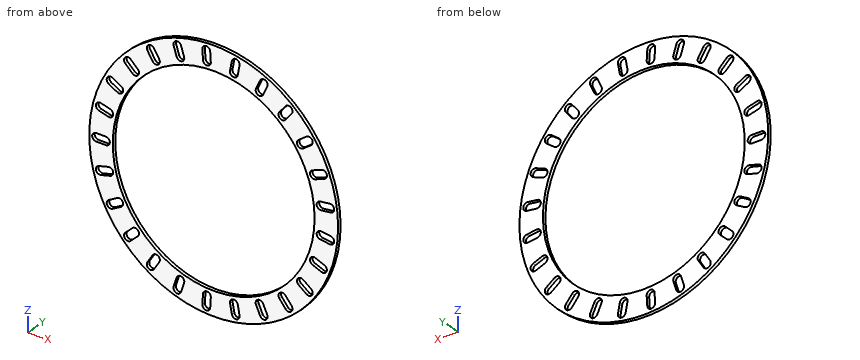
from build123d import *

# Parameters (mm, degrees)
SKETCH1_R           = 31.77
SKETCH1_R_2         = 25.77
BOSS_EXTRUDE1_DEPTH = 0.85
CUT_EXTRUDE1_DEPTH  = 1.85
CIRPATTERN1_COUNT   = 25


with BuildPart() as part:
    # Sketch1 → Boss-Extrude1 (new body)
    with BuildSketch(Plane(origin=(0, 0, 0), x_dir=(1, 0, 0), z_dir=(0, 1, 0))):
        Circle(SKETCH1_R)
        Circle(SKETCH1_R_2, mode=Mode.SUBTRACT)
    extrude(amount=BOSS_EXTRUDE1_DEPTH)

    # Sketch3 → Cut-Extrude1 (cut, through all)
    with BuildSketch(Plane(origin=(0, 0.85, 0), x_dir=(1, 0, 0), z_dir=(0, 1, 0))):
        with BuildLine():
            Line((-30.02, 1), (-27.52, 1))
            ThreePointArc((-27.52, 1), (-26.52, 0), (-27.52, -1))
            Line((-27.52, -1), (-30.02, -1))
            ThreePointArc((-30.02, -1), (-31.02, 0), (-30.02, 1))
        make_face()
    cut_extrude1 = extrude(amount=-CUT_EXTRUDE1_DEPTH, mode=Mode.SUBTRACT)

    # CirPattern1: Cut-Extrude1 ×25 about axis
    cirpattern1_axis = Axis((0, 0, 0), (0, 1, 0))
    for i in range(1, CIRPATTERN1_COUNT):
        add(cut_extrude1.rotate(cirpattern1_axis, i * 360 / CIRPATTERN1_COUNT), mode=Mode.SUBTRACT)


solid = part.part
The listing builds one solid part. Answer for the finished solid, in the listing's coordinates (mm). Give positions to 0.01 mm unless a question says otherwise; leave off trailing zeros. Write each loop counter-clockwise with the first axis right and the second up, starting at its lowest first coordinate (ties: lowest second). Pieces come first, ordered by that corner, then holes. Notation, with made-up numbers: (-29, -23) -> (3, -23) arc R20 ccw to (3, -19) -> close; hole circle Ø3 at (-16, 88). An arc over 180 degrees is marked (long way). Use a Markdown table: item, result.
(1) Section C-C, the plane y = 0.6 is taken. Give the number of separate pieces and of enclosed holes in the cut face, then the cut area to 3 significant figures.
Return value:
| item | result |
|---|---|
| separate pieces | 1 |
| enclosed holes | 26 |
| area | 881 mm2 |
(2) Section D-D, the plane x = -11 is taken. Determine the outline of the cut face in (y, z).
Return value:
| item | result |
|---|---|
| outline | (0, -29.8) -> (0.85, -29.8) -> (0.85, -23.3) -> (0, -23.3) -> close; (0, 23.3) -> (0.85, 23.3) -> (0.85, 29.8) -> (0, 29.8) -> close |
(3) Section A-A, the plane z = 0 is taken. Determine the outline of the cut face in (x, y), then the cut area to 4 significant figures.
Return value:
| item | result |
|---|---|
| outline | (-31.77, 0) -> (-31.02, 0) -> (-31.02, 0.85) -> (-31.77, 0.85) -> close; (-26.52, 0) -> (-25.77, 0) -> (-25.77, 0.85) -> (-26.52, 0.85) -> close; (25.77, 0) -> (31.77, 0) -> (31.77, 0.85) -> (25.77, 0.85) -> close |
| area | 6.375 mm2 |
(4) Find the intervals of material crossed by probe 1 along X at (y, z) = (0.25, 0); probe 2 along Z at (x, y) = (0, 0.45); probe 3 along X at (y, z) = (0.45, 23), in increasing order. Write a range as from..to.
Return value:
| item | result |
|---|---|
| probe 1 | -31.77..-31.02, -26.52..-25.77, 25.77..31.77 |
| probe 2 | -31.77..-25.77, 25.77..31.77 |
| probe 3 | -21.92..-15.78, -13.77..-11.62, 11.62..17.73, 20.13..21.92 |
(5) Section B-B, the plane x = 0 is taken. Determine the outline of the cut face in (y, z), then the cut area to 3 significant figures.
Return value:
| item | result |
|---|---|
| outline | (0, -31.77) -> (0.85, -31.77) -> (0.85, -25.77) -> (0, -25.77) -> close; (0, 25.77) -> (0.85, 25.77) -> (0.85, 31.77) -> (0, 31.77) -> close |
| area | 10.2 mm2 |
